```python
from build123d import *

# Parameters (mm, degrees)
SKETCH_1_R               = 29
EXTRUDE_1_DEPTH          = 5
HOLE_WIZARD_1_D          = 3.5
HOLE_WIZARD_2_D          = 23
EXTRUDE_3_DEPTH          = 65
SKETCH_9_W               = 1
SKETCH_9_H               = 5
CUT_EXTRUDE_1_DEPTH      = 10
SKETCH_10_W              = 3
SKETCH_10_H              = 65
EXTRUDE_5_DEPTH          = 10
HOLE_WIZARD_3_D          = 3.5
CUT_EXTRUDE_2_REACH      = 97.355
SKETCH_16_W              = 20
SKETCH_16_H              = 3
EXTRUDE_START            = -65
EXTRUDE_6_DEPTH          = 65
HOLE_WIZARD_4_D          = 3.5
SKETCH_22_W              = 12
SKETCH_22_H              = 6
EXTRUDE_7_DEPTH          = 3
EXTRUDE_8_DEPTH          = 8
HOLE_WIZARD_5_D          = 7
HOLE_WIZARD_5_DEPTH      = 3
SKETCH_27_W              = 5
SKETCH_27_H              = 3.5
CUT_EXTRUDE_3_DEPTH      = 70.598725899
CUT_EXTRUDE_4_REACH      = 94.289
SKETCH_28_W              = 3
SKETCH_28_H              = 3.5
SKETCH_29_R              = 3.5
EXTRUDE_9_DEPTH          = 18
HOLE_WIZARD_6_D          = 10.4
HOLE_WIZARD_6_DEPTH      = 18
SKETCH_32_W              = 26
SKETCH_32_H              = 5
EXTRUDE_10_DEPTH         = 9
CUT_EXTRUDE_5_REACH      = 88.897
EXTRUDE_11_DEPTH         = 65
CUT_EXTRUDE_6_REACH      = 94.404
CUT_EXTRUDE_6_END_RADIUS = 29


with BuildPart() as part:
    # 草图1 → 凸台-拉伸1 (new body)
    with BuildSketch(Plane.XY):
        Circle(SKETCH_1_R)
    extrude(amount=EXTRUDE_1_DEPTH)

    # 孔1 (through all)
    with Locations(Plane.XY.offset(5)):
        with Locations((0, 20), (-17.320508076, -10), (17.320508076, -10)):
            Hole(HOLE_WIZARD_1_D / 2)

    # 孔2 (through all)
    with Locations(Plane.XY.offset(5)):
        with Locations((0, 0)):
            Hole(HOLE_WIZARD_2_D / 2)

    # 草图7 → 凸台-拉伸3 (add)
    with BuildSketch(Plane.XY.offset(5)):
        with BuildLine():
            Line((-28.892040426, 2.5), (-28.892040426, -2.5))
            Line((-28.892040426, -2.5), (-11.22497216, -2.5))
            ThreePointArc((-11.22497216, -2.5), (-11.5, 0), (-11.22497216, 2.5))
            Line((-11.22497216, 2.5), (-28.892040426, 2.5))
        make_face()
    extrude(amount=EXTRUDE_3_DEPTH)

    # 草图9 → 切除-拉伸1 (cut)
    with BuildSketch(Plane.XY.offset(5)):
        with Locations((-29.392040426, 0)):
            Rectangle(SKETCH_9_W, SKETCH_9_H)
    extrude(amount=-CUT_EXTRUDE_1_DEPTH, mode=Mode.SUBTRACT)

    # 草图10 → 凸台-拉伸5 (add)
    with BuildSketch(Plane(origin=(0, 2.5, 0), x_dir=(1, 0, 0), z_dir=(0, 1, 0))):
        with Locations((-27.392040426, -37.5)):
            Rectangle(SKETCH_10_W, SKETCH_10_H)
    extrude(amount=EXTRUDE_5_DEPTH)

    # 孔3 (through all)
    with Locations(Plane.ZY.offset(28.892040426)):
        with Locations((10, 7.5), (64.4, 7.5)):
            Hole(HOLE_WIZARD_3_D / 2)

    # 草图16 → 切除-拉伸2 (cut, up to next)
    with BuildSketch(Plane.ZY.offset(28.892040426), mode=Mode.PRIVATE) as cut_extrude_2_sk1:
        with Locations((35, 11)):
            Rectangle(SKETCH_16_W, SKETCH_16_H)
    cut_extrude_2_tool1 = extrude(cut_extrude_2_sk1.sketch, amount=-CUT_EXTRUDE_2_REACH, mode=Mode.PRIVATE) & part.part
    add(cut_extrude_2_tool1.solids().sort_by_distance((-28.89204, 11, 35))[0], mode=Mode.SUBTRACT)

    # 草图20 → 凸台-拉伸6 (add)
    with BuildSketch(Plane.XY.offset(70).offset(EXTRUDE_START)):
        with BuildLine():
            Line((-11.22497216, 2.5), (-11.22497216, -2.5))
            ThreePointArc((-11.22497216, -2.5), (-11.5, 0), (-11.22497216, 2.5))
        make_face()
    extrude(amount=EXTRUDE_6_DEPTH)

    # 孔4 (through all)
    with Locations(Plane.ZY.offset(28.892040426)):
        with Locations((25, 0), (45, 0)):
            Hole(HOLE_WIZARD_4_D / 2)

    # 草图22 → 凸台-拉伸7 (add)
    with BuildSketch(Plane.ZY.offset(28.892040426)):
        with Locations((57.4, 15.5)):
            Rectangle(SKETCH_22_W, SKETCH_22_H)
    extrude(amount=-EXTRUDE_7_DEPTH)

    # 草图23 → 凸台-拉伸8 (add)
    with BuildSketch(Plane.ZY.offset(28.892040426)):
        Polygon((51.4, 6.5), (60.801923789, 6.5), (63.4, 11), (63.4, 12.5), (63.4, 18.5), (51.4, 18.5), (51.4, 12.5), align=None)
    extrude(amount=EXTRUDE_8_DEPTH)

    # 孔5
    with Locations(Plane.ZY.offset(36.892040426)):
        with Locations((57.4, 12.5)):
            Hole(HOLE_WIZARD_5_D / 2, depth=HOLE_WIZARD_5_DEPTH)

    # 草图27 → 切除-拉伸3 (cut, through all)
    with BuildSketch(Plane(origin=(0, 0, 51.4), x_dir=(-1, 0, 0), z_dir=(0, 0, -1))):
        with Locations((31.392040426, 14.25)):
            Rectangle(SKETCH_27_W, SKETCH_27_H)
        with Locations((31.392040426, 10.75)):
            Rectangle(SKETCH_27_W, SKETCH_27_H)
    extrude(amount=-CUT_EXTRUDE_3_DEPTH, mode=Mode.SUBTRACT)

    # 草图28 → 切除-拉伸4 (cut, up to next)
    with BuildSketch(Plane(origin=(0, 18.5, 0), x_dir=(1, 0, 0), z_dir=(0, 1, 0)), mode=Mode.PRIVATE) as cut_extrude_4_sk1:
        with Locations((-32.392040426, -59.15)):
            Rectangle(SKETCH_28_W, SKETCH_28_H)
    cut_extrude_4_tool1 = extrude(cut_extrude_4_sk1.sketch, amount=-CUT_EXTRUDE_4_REACH, mode=Mode.PRIVATE) & part.part
    # 草图28 → 切除-拉伸4 (cut, up to next)
    with BuildSketch(Plane(origin=(0, 18.5, 0), x_dir=(1, 0, 0), z_dir=(0, 1, 0)), mode=Mode.PRIVATE) as cut_extrude_4_sk2:
        with Locations((-32.392040426, -55.65)):
            Rectangle(SKETCH_28_W, SKETCH_28_H)
    cut_extrude_4_tool2 = extrude(cut_extrude_4_sk2.sketch, amount=-CUT_EXTRUDE_4_REACH, mode=Mode.PRIVATE) & part.part
    add(cut_extrude_4_tool1.solids().sort_by_distance((-32.39204, 18.5, 59.15))[0], mode=Mode.SUBTRACT)
    add(cut_extrude_4_tool2.solids().sort_by_distance((-32.39204, 18.5, 55.65))[0], mode=Mode.SUBTRACT)

    # 草图29 → 凸台-拉伸9 (add)
    # profile 1 of 2: a face of its own
    with BuildSketch(Plane.ZY.offset(36.892040426)):
        Polygon((60.801923789, 6.5), (63.4, 11), (63.4, 18.5), (51.4, 18.5), (51.4, 6.5), align=None)
        with Locations((57.4, 12.5)):
            Circle(SKETCH_29_R, mode=Mode.SUBTRACT)
    # profile 2 of 2: a face of its own
    with BuildSketch(Plane.ZY.offset(36.892040426)):
        with Locations((57.4, 12.5)):
            Circle(SKETCH_29_R)
    extrude(amount=EXTRUDE_9_DEPTH)

    # 孔6
    with Locations(Plane.ZY.offset(54.892040426)):
        with Locations((57.4, 12.5)):
            Hole(HOLE_WIZARD_6_D / 2, depth=HOLE_WIZARD_6_DEPTH)

    # 草图32 → 凸台-拉伸10 (add)
    with BuildSketch(Plane.XZ.offset(-6.5)):
        with Locations((-41.892040426, 58.301923789)):
            Rectangle(SKETCH_32_W, SKETCH_32_H)
    extrude(amount=EXTRUDE_10_DEPTH)

    # 草图33 → 切除-拉伸5 (cut, up to next)
    with BuildSketch(Plane.XY.offset(60.801923789), mode=Mode.PRIVATE) as cut_extrude_5_sk1:
        Polygon((-54.892040426, 6.5), (-28.892040426, -2.5), (-54.892040426, -2.5), align=None)
    cut_extrude_5_tool1 = extrude(cut_extrude_5_sk1.sketch, amount=-CUT_EXTRUDE_5_REACH, mode=Mode.PRIVATE) & part.part
    add(cut_extrude_5_tool1.solids().sort_by_distance((-46.225374, 0.5, 60.801924))[0], mode=Mode.SUBTRACT)

    # 草图34 → 凸台-拉伸11 (add)
    with BuildSketch(Plane.XY.offset(5)):
        with BuildLine():
            Line((-23.892040426, -16.436861144), (-23.892040426, -2.5))
            Line((-23.892040426, -2.5), (-28.892040426, -2.5))
            ThreePointArc((-28.892040426, -2.5), (-27.296498356, -9.792914658), (-23.892040426, -16.436861144))
        make_face()
    extrude(amount=EXTRUDE_11_DEPTH)

    # 切除-拉伸6: up to this cylinder (the profile starts inside it)
    cut_extrude_6_end = Plane(origin=(0, 0, 45.61427), z_dir=(0, 0, -1)) * Cylinder(CUT_EXTRUDE_6_END_RADIUS, 247.808, mode=Mode.PRIVATE)
    # 草图35 → 切除-拉伸6 (cut, up to the surface)
    with BuildSketch(Plane(origin=(-23.892040426, 0, 0), x_dir=(0, 0, -1), z_dir=(1, 0, 0)), mode=Mode.PRIVATE) as cut_extrude_6_sk1:
        Polygon((-70, -2.5), (-5, -14.436861144), (-5, -16.436861144), (-70, -16.436861144), align=None)
    cut_extrude_6_tool1 = extrude(cut_extrude_6_sk1.sketch, amount=-CUT_EXTRUDE_6_REACH, mode=Mode.PRIVATE) & cut_extrude_6_end
    add(cut_extrude_6_tool1.solids().sort_by_distance((-23.89204, -11.707577, 45.61427))[0], mode=Mode.SUBTRACT)


solid = part.part
```
Can you work these out from the model? Positions are in its coordinate system, mm. A direction names the side the tool comes from. Give positions to 0.01 mm unless a question says otherwise; leave off trailing zeros. Loops run counter-clockwise (first coordinate to the right, second up) from the corner with the lowest first, then second, coordinate; pieces in that order, holes last. Notation, with made-up numbers: M 0,66.25 L 20,66.25 A5 ccw 20,70.25 Z; hole C -31.75,2.25 d1. An arc over 180 degrees is marked long. Use CSV: the item, a comma, the result in double quotes. Start each with the question number.
1. If we mould it in two halves opening along Z, with no side actions, what happens to faces 5 (the face through (-27, 9.5, 35)), 6 (the face through (13, 0, 5)), 7 (the face through (-54.892, 18, 57)), 8 (the face through (-28, 10, 5))? For each: released by +Z, released by -Z, zero draft, split by the parting line, or undercut.
2. For P1, Ø3.5, axis at x = -27, z = 37, coming from the +Y side; P2, Ø5.5, axis at y = -1, z = 52.5, coming from the +X side (3 decimals); P3, Ø16, axis at x = -20, z = 22, coming from the +Y side; P4, Ø6, axis at y = -12.5, z = 47.5, coming from the -X side, each with a flat end and sliding along its axis, tell me the tip position at first contact or that it passes through.
3. Imagine slicing it at C-C, the plane y = -10. Write out the boundary of the cut face in (x, z), plus the area to 3 significant figures.
4. Imagine slicing it at A-A, the plane x = 0. Write out the boundary of the cut face in (y, z).
5. If I drill on L1, parallel to Y at x = 0, z = 2.7; L2, parallel to X at y = 0, z = 1.95; L3, parallel to Z at x = 10.5, y = 20.5, over which ranges is the centre line in solid material (lowest first)?
6. On a 3-axis mill with a long thin cutter (end or side, diameter ignored), from which of +Z, -Z, +X, -X, +Y, -Y can I reach the whole of each face in a straight line? I mean faces 1 (the face through (-45.766, 12.729, 62.595)), 2 (the face through (-32, 17, 53.9)), 3 (the face through (-18, -2.5, 38)), 4 (the face through (-33.892, 16, 56)). Say none if no direction works.
7. Imagine slicing it at D-D, the plane z = 21. Write out the boundary of the cut face in (x, y), plus the area to 3 significant figures.
8. Imagine slicing it at B-B, the plane z = 64.4. Write out the boundary of the cut face in (x, y).
Response values:
1,face 5,"undercut"
1,face 6,"released by +Z"
1,face 7,"zero draft"
1,face 8,"released by -Z"
2,P1,"y = 9.5"
2,P2,"x = -11.225"
2,P3,"y = 12.5"
2,P4,"through"
3,outline,"M -27.22,0 L -19.07,0 L -19.07,5 L -23.89,5 L -23.89,29.16 L -27.22,29.16 Z; M -15.57,0 L -5.68,0 L -5.68,5 L -15.57,5 Z; M 5.68,0 L 15.57,0 L 15.57,5 L 5.68,5 Z; M 19.07,0 L 27.22,0 L 27.22,5 L 19.07,5 Z"
3,area,"261 mm^2"
4,outline,"M -29,0 L -11.5,0 L -11.5,5 L -29,5 Z; M 11.5,0 L 18.25,0 L 18.25,5 L 11.5,5 Z; M 21.75,0 L 29,0 L 29,5 L 21.75,5 Z"
5,L1,"-29 to -11.5, 11.5 to 18.25, 21.75 to 29"
5,L2,"-28.89 to -11.5, 11.5 to 29"
5,L3,"0 to 5"
6,face 1,"-X"
6,face 2,"+Y"
6,face 3,"+Z, +X, -Y"
6,face 4,"none"
7,outline,"M -28.89,-2.5 A29 ccw -26.62,-11.5 L -23.89,-11.5 L -23.89,-2.5 L -11.22,-2.5 L -11.22,2.5 L -25.89,2.5 L -25.89,12.5 L -28.89,12.5 Z"
7,area,"155 mm^2"
8,outline,"M -28.89,-2.5 A29 ccw -28.78,-3.53 L -23.89,-3.53 L -23.89,-2.5 L -11.22,-2.5 L -11.22,2.5 L -25.89,2.5 L -25.89,5.75 L -28.89,5.75 Z; M -28.89,9.25 L -25.89,9.25 L -25.89,12.5 L -28.89,12.5 Z"
